The figure shows three views and two pictorial views of one solid part (mm, origin at its lowest corner). Answer the questions. A direction names the side the tool comes from. Coordinates: 2 decimals unless noted, no trailing zeros. Order: outer loops, then holes, each group sorted by start corner. A loop starts at its lowest first (then second) coordinate and runs counter-clockwise, first axis right, second up. Notation, with made-up numbers: (-5, 15.25) -> (0, 15.25) arc R8 cw to (0, 21.25) -> close; hole circle Ø8 at (15.25, -39.5). An arc over 180 degrees is marked (long way). Write item = value, one per line. Start each with the question number.
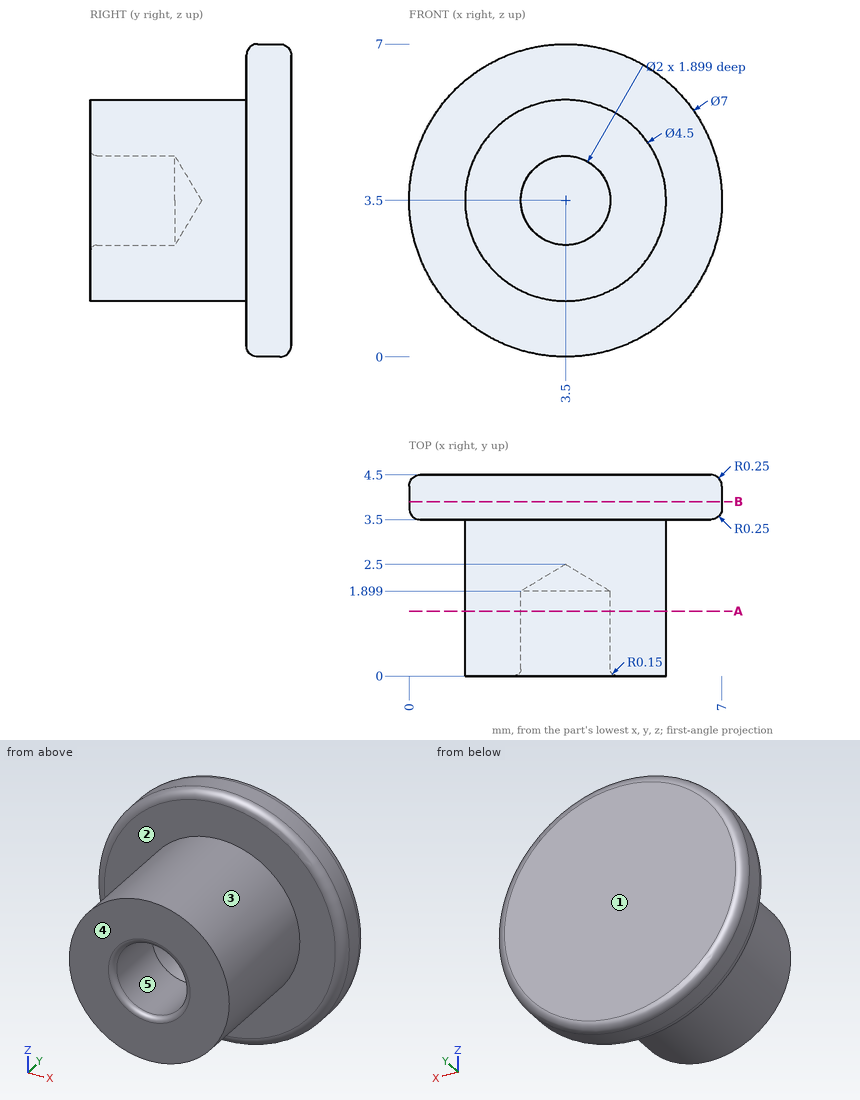
Item 1: Consider probe 1 along Z at (x, y) = (3.25, 2.25) (1 decimal); probe 2 along X at (y, z) = (1.15, 2.75); probe 3 along Y at (x, z) = (6.75, 3.5). Determine where each line is inside the solid, lowest interval first.
Item 2: For a pull along Z with two mould halves and no side action, classify the marked faces 3, 4 and 5 as pulls with the +Z half, pulls with the -Z half, needs draft (parallel to the pull), parting line crosses it, or undercut.
Item 3: Section A-A, the plane y = 1.45 is taken. Give the vertices of the cut face in (x, z).
Item 4: Section B-B, the plane y = 3.9 is taken. Give the vertices of the cut face in (x, z).
Item 5: Which of the six approach directions +Z, -Z, +X, -X, +Y, -Y give full straight-line access (tool end or side, diameter ignored) to the marked faces 1 and 2?
Item 6: This flat-tipped pin is pushed along its axis until it touches: pin 1 (1.5 mm diameter, centred on y = 3.5, z = 2.5, fed in from -X). Where does it stop, or does it pass through?
A:
q1.probe_1 = 1.3 to 3.2, 3.8 to 5.7
q1.probe_2 = 1.38 to 2.84, 4.16 to 5.62
q1.probe_3 = 3.5 to 4.5
q2.face_3 = parting line crosses it
q2.face_4 = needs draft
q2.face_5 = undercut
q3.outline = circle Ø4.5 at (3.5, 3.5); hole circle Ø2 at (3.5, 3.5)
q4.outline = circle Ø7 at (3.5, 3.5)
q5.face_1 = +Z, -Z, +X, -X, +Y
q5.face_2 = -Y
q6.pin_1 = 0.01
